Can you work these out from the model? Positions are in its coordinate system, mm. A direction names the side the tool comes from. Give positions to 0.01 mm unless a question says otherwise; leave off trailing zeros. Order: outer loops, then holes, each group sorted by start corner. A loop starts at its lowest first (then second) coordinate and runs counter-clockwise, first axis right, second up. Notation, with made-up numbers: M 33.5,52 L 82.5,52 A20 cw 82.5,76 Z; hole C -40,64 d5. An arc over 180 degrees is marked long. Use a Markdown table: item, result. Add a question column.
from build123d import *

# Parameters (mm, degrees)
F0_W      = 24.9936
F0_H      = 24.9936
F1_DEPTH  = 24.9936
F2_R      = 11
F3_DEPTH  = 8
F4_R      = 1.524
F6_DEPTH  = 10
F8_DEPTH  = 6
F9_R      = 1.5875
F10_DEPTH = 11.684
F11_R     = 2.54
F12_DEPTH = 25.4


with BuildPart() as f1:
    # F0 (on Top) → F1 (new body)
    with BuildSketch(Plane.XY):
        Rectangle(F0_W, F0_H)
    extrude(amount=F1_DEPTH)

    # F2 (on face) → F3 (join)
    with BuildSketch(Plane.XY.offset(24.9936)):
        Circle(F2_R)
    extrude(amount=F3_DEPTH)

    # F4
    f4_edges = [f1.edges().sort_by_distance(p)[0] for p in [
        (-11, 0, 32.9936),
    ]]
    fillet(f4_edges, radius=F4_R)

    # F5 (on face) → F6 (cut)
    with BuildSketch(Plane.XY.offset(32.9936)):
        with BuildLine():
            Line((-1.65, 0), (-1.65, -1.299038))
            ThreePointArc((-1.65, -1.299038), (0.687386, -1.984313), (2.1, 0))
            Line((2.1, 0), (-1.65, 0))
        make_face()
        with BuildLine():
            Line((-1.65, 0), (2.1, 0))
            ThreePointArc((2.1, 0), (0.687386, 1.984313), (-1.65, 1.299038))
            Line((-1.65, 1.299038), (-1.65, 0))
        make_face()
    extrude(amount=-F6_DEPTH, mode=Mode.SUBTRACT)

    # F7 (on face) → F8 (cut)
    with BuildSketch(Plane.XY.offset(32.9936)):
        Polygon((-4.15, 0), (-4.15, 3), (-6.65, 3), (-6.65, -3), (-4.15, -3), align=None)
    extrude(amount=-F8_DEPTH, mode=Mode.SUBTRACT)

    # F9 (on face) → F10 (cut)
    with BuildSketch(Plane(origin=(-12.4968, 0, 0), x_dir=(0, -1, 0), z_dir=(-1, 0, 0))):
        with Locations((0, 28.492712)):
            Circle(F9_R)
    extrude(amount=-F10_DEPTH, mode=Mode.SUBTRACT)

    # F11 (on face) → F12 (cut)
    with BuildSketch(Plane.YZ.offset(12.4968)):
        with Locations((-6.5024, 16.1036)):
            Circle(F11_R)
        with Locations((6.5024, 16.1036)):
            Circle(F11_R)
    extrude(amount=-F12_DEPTH, mode=Mode.SUBTRACT)


solid = f1.part
1. Will these pins go through, and if not, where does the flat tip stop? pin 1 (3 mm diameter, centred on y = 0, z = 31, fed in from +X); pin 2 (1.2 mm diameter, centred on x = -6, z = 29.5, fed in from -Y); pin 3 (4 mm diameter, centred on y = -6.5, z = 16.1, fed in from -X); pin 4 (0.7 mm diameter, centred on x = -5, y = 1.5, fed in from +Z).
2. If we section it at C-C, the plane x = 2.5: State how many separate pieces and enclosed holes the cut face has, then the cut area to 3 significant figures.
3. I need wall thicknesses on L1, parallel to Y at x = 7.5, z = 16; L2, parallel to Y at x = 5.25, z = 17.5; L3, parallel to Z at x = 5.75, y = 10. Which ranges of each line are inside material? Lowest first, please. Write a range as [from, to].
4. On a 3-axis mill with a long thin cutter (end or side, diameter ignored), from which of +Z, -Z, +X, -X, +Y, -Y can I reach the whole of each face in a straight line? I mean faces 4 (the face through (-5, -3, 30)), 5 (the face through (12.497, 0, 12)). Say none if no direction works.
5. If we section it at B-B, the plane x = 0: List the corners of the cut face in (y, z) for me.
6. If we section it at A-A, the plane z = 26.5: List the corners of the cut face in (x, y) for me.
7. We'd pull the mould along Z, two halves only. Please class faces 1 (the face through (0, 0, 0)), 2 (the face through (0, -12.497, 12)), 3 (the face through (-6.255, 0.344, 26.943)): +Z half, -Z half, draft (parallel to the pull), parting line (faces both ways), or undercut.
Geometry results:
| question | item | result |
|---|---|---|
| 1 | pin 1 | stops at x = 11 |
| 1 | pin 2 | stops at y = -9.58 |
| 1 | pin 3 | passes through |
| 1 | pin 4 | stops at z = 26.99 |
| 2 | separate pieces | 1 |
| 2 | enclosed holes | 2 |
| 2 | area | 755 mm^2 |
| 3 | L1 | y = [-12.5, -9.04], [-3.96, 3.96], [9.04, 12.5] |
| 3 | L2 | y = [-12.5, -8.62], [-4.38, 4.38], [8.62, 12.5] |
| 3 | L3 | z = [0, 24.99] |
| 4 | face 4 | +Z |
| 4 | face 5 | +Z, -Z, +X, +Y, -Y |
| 5 | outline | M -12.5,0 L 12.5,0 L 12.5,24.99 L 11,24.99 L 11,31.47 A1.52 ccw 9.48,32.99 L 2.1,32.99 L 2.1,22.99 L -2.1,22.99 L -2.1,32.99 L -9.48,32.99 A1.52 ccw -11,31.47 L -11,24.99 L -12.5,24.99 Z; hole C -6.5,16.1 d5.08; hole C 6.5,16.1 d5.08 |
| 6 | outline | C 0,0 d22; hole M -1.65,-1.3 A2.1 ccw 2.1,0 A2.1 ccw -1.65,1.3 Z |
| 7 | face 1 | -Z half |
| 7 | face 2 | draft |
| 7 | face 3 | undercut |
